The figure shows three views and two pictorial views of one solid part (mm, origin at its lowest corner). Answer the questions. A direction names the side the tool comes from. Round coordinates to 2 decimals unless told otherwise and drop trailing zeros. Loops run counter-clockwise (first coordinate to the right, second up) from the corner with the lowest first, then second, coordinate; pieces in that order, holes last. Notation, with made-up numbers: (6.5, 36.25) -> (30.5, 36.25) arc R27 cw to (30.5, 57.25) -> close; hole circle Ø3 at (-28, 43). An arc over 180 degrees is marked (long way). Put each result on its own line as item: value.
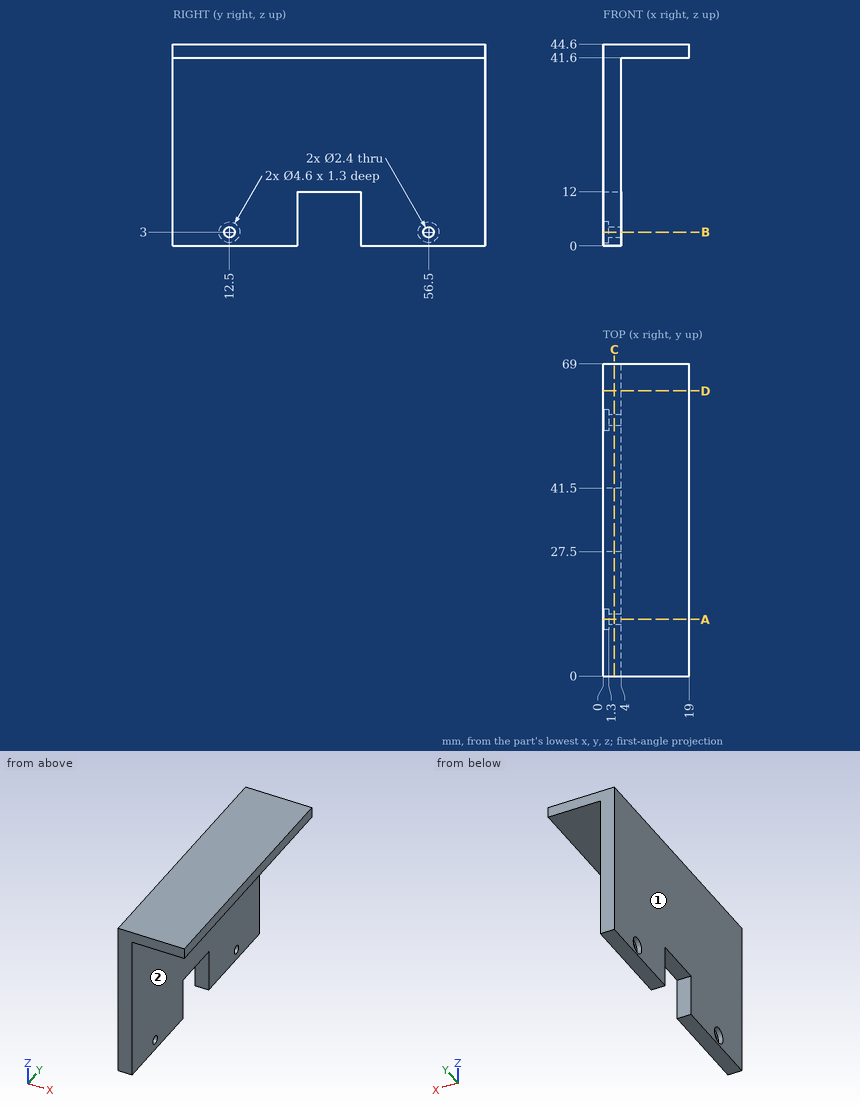
Item 1: The part is cut by section A-A (y = 12.5). Determine the outline of the cut face in (x, z), then the cut area to 3 significant figures.
Derived:
outline: (0, 0) -> (4, 0) -> (4, 1.8) -> (1.3, 1.8) -> (1.3, 0.7) -> (0, 0.7) -> close; (0, 5.3) -> (1.3, 5.3) -> (1.3, 4.2) -> (4, 4.2) -> (4, 41.6) -> (19, 41.6) -> (19, 44.6) -> (0, 44.6) -> close
area: 211 mm^2
Item 2: The part is cut by section D-D (y = 63). Determine the outline of the cut face in (x, z), then the cut area to 3 significant figures.
Derived:
outline: (0, 0) -> (4, 0) -> (4, 41.6) -> (19, 41.6) -> (19, 44.6) -> (0, 44.6) -> close
area: 223 mm^2
Item 3: Flat-ended cylindrical pins translate along their axes: pin 1 Ø1.2 at (x, y) = (2, 32.5) entering from -Z; pin 2 Ø3 at (y, z) = (8.5, 14.5) entering from +X; pin 3 Ø1.4 at (y, z) = (12, 3.5) entering from -X. Find the tip coordinate at first contact, or state that the pin passes through.
Derived:
pin 1: stops at z = 12
pin 2: stops at x = 4
pin 3: stops at x = 1.3
Item 4: The part is cut by section B-B (z = 3). Determine the outline of the cut face in (x, y), then the cut area to 3 significant figures.
Derived:
outline: (0, 0) -> (4, 0) -> (4, 11.3) -> (1.3, 11.3) -> (1.3, 10.2) -> (0, 10.2) -> close; (0, 14.8) -> (1.3, 14.8) -> (1.3, 13.7) -> (4, 13.7) -> (4, 27.5) -> (0, 27.5) -> close; (0, 41.5) -> (4, 41.5) -> (4, 55.3) -> (1.3, 55.3) -> (1.3, 54.2) -> (0, 54.2) -> close; (0, 58.8) -> (1.3, 58.8) -> (1.3, 57.7) -> (4, 57.7) -> (4, 69) -> (0, 69) -> close
area: 195 mm^2
Item 5: Which of the six approach directions +Z, -Z, +X, -X, +Y, -Y give full straight-line access (tool end or side, diameter ignored) to the marked faces 1 and 2?
Derived:
face 1: +Z, -Z, -X, +Y, -Y
face 2: -Z, +X, +Y, -Y
Item 6: The part is cut by section C-C (x = 2.5). Determine the outline of the cut face in (y, z), then the cut area to 3 significant figures.
Derived:
outline: (0, 0) -> (27.5, 0) -> (27.5, 12) -> (41.5, 12) -> (41.5, 0) -> (69, 0) -> (69, 44.6) -> (0, 44.6) -> close; hole circle Ø2.4 at (12.5, 3); hole circle Ø2.4 at (56.5, 3)
area: 2,900 mm^2
Item 7: Find the intervals of material crossed by line 1 along Y through (x, z) = (2.5, 3); line 2 along Y through (x, z) = (0.75, 3); line 3 along Z through (x, y) = (0.7, 56.5), in increasing order.
Derived:
line 1: y = 0 to 11.3, 13.7 to 27.5, 41.5 to 55.3, 57.7 to 69
line 2: y = 0 to 10.2, 14.8 to 27.5, 41.5 to 54.2, 58.8 to 69
line 3: z = 0 to 0.7, 5.3 to 44.6
